from build123d import *

# Parameters (mm, degrees)
F0_W     = 15
F0_H     = 15
F1_DEPTH = 15
F4_ANGLE = 45
F5_ANGLE = 45


with BuildPart() as f1:
    # F0 (on Front) → F1 (new body)
    with BuildSketch(Plane.XZ):
        with Locations((-7.5, 7.5)):
            Rectangle(F0_W, F0_H)
    extrude(amount=F1_DEPTH)


with BuildPart() as f1_1:
    # F4: moved
    add(f1.part.rotate(Axis((-5.703268, 0, 0), (-1, 0, 0)), F4_ANGLE))


with BuildPart() as f1_2:
    # F5: moved
    add(f1_1.part.rotate(Axis((0, 0, 2.941495), (0, 0, -1)), F5_ANGLE))


solid = f1_2.part
Geometry check sheet. Reference: the model listing, model coordinates, mm. Give positions to 0.01 mm unless a question says otherwise; leave off trailing zeros. Write each loop counter-clockwise with the first axis right and the second up, starting at its lowest first coordinate (ties: lowest second). Pieces come first, ordered by that corner, then holes.
1) Go/stop test with flat-tipped pins: pin 1 Ø1 at (y, z) = (-2, 13) entering from +X; pin 2 Ø1 at (x, y) = (3.5, 10) entering from -Z; pin 3 Ø3 at (x, y) = (-7, -2) entering from +Z. Record where each tip stops, or that it passes through.
Values follow:
pin 1: stops at x = -1.5
pin 2: stops at z = 9.05
pin 3: stops at z = 16.35
2) Cross-section at A-A (y = 1.75). Record the boundary of the cut face in (x, z).
Values follow:
outline: (-16.75, 10.61) - (-1.75, 0) - (1.75, 2.47) - (1.75, 18.74) - (-1.75, 21.21) - close
3) Cross-section at B-B (x = -7). Record the boundary of the cut face in (y, z).
Values follow:
outline: (-7, 9.9) - (7, 0) - (14.21, 5.1) - (14.21, 16.11) - (7, 21.21) - (-7, 11.31) - close
4) Cross-section at C-C (z = 12.75). Record the boundary of the cut face in (x, y), plus the area to 3 significant figures.
Values follow:
outline: (-16.59, 4.62) - (-5.98, -5.98) - (5.98, 5.98) - (-4.62, 16.59) - close
area: 254 mm2
5) Thickness scan on line 1 (X direction, y = 3, z = 12); line 2 (Y direction, x = -2.5, z = 1); line 3 (X direction, y = 9.5, z = 19.5). Record the ranges inside material, lowest first.
Values follow:
line 1: x = -16.03 to 3
line 2: y = 1.09 to 3.91
line 3: x = -11.71 to -7.08
6) Cross-section at D-D (z = 19.5). Record the boundary of the cut face in (x, y).
Values follow:
outline: (-11.82, 9.4) - (-1.21, -1.21) - (1.21, 1.21) - (-9.4, 11.82) - close
